from build123d import *

# Parameters (mm, degrees)
SKETCH1_R           = 61.3
BOSS_EXTRUDE1_DEPTH = 1.65
SKETCH2_R           = 55.89
BOSS_EXTRUDE2_DEPTH = 32.735
SKETCH3_R           = 50.86
CUT_EXTRUDE1_DEPTH  = 14.35
SKETCH5_R           = 19.45
BOSS_EXTRUDE3_DEPTH = 0.2
SCALE2_SCALE        = 0.5


with BuildPart() as part:
    # Sketch1 → Boss-Extrude1 (new body)
    with BuildSketch(Plane(origin=(0, 0, 0), x_dir=(1, 0, 0), z_dir=(0, 1, 0))):
        Circle(SKETCH1_R)
    extrude(amount=BOSS_EXTRUDE1_DEPTH)

    # Sketch2 → Boss-Extrude2 (add)
    with BuildSketch(Plane(origin=(0, 1.65, 0), x_dir=(1, 0, 0), z_dir=(0, 1, 0))):
        Circle(SKETCH2_R)
    extrude(amount=BOSS_EXTRUDE2_DEPTH)

    # Sketch3 → Cut-Extrude1 (cut)
    with BuildSketch(Plane.XZ):
        Circle(SKETCH3_R)
    extrude(amount=-CUT_EXTRUDE1_DEPTH, mode=Mode.SUBTRACT)

    # Sketch5 → Boss-Extrude3 (add)
    with BuildSketch(Plane(origin=(0, 34.385, 0), x_dir=(1, 0, 0), z_dir=(0, 1, 0))):
        Circle(SKETCH5_R)
    extrude(amount=BOSS_EXTRUDE3_DEPTH)


with BuildPart() as part_1:
    # Scale2: scaled about (0, 22.178245993, 0)
    add(part.part.scale(SCALE2_SCALE).moved(Location((0, 11.089122997, 0))))


solid = part_1.part
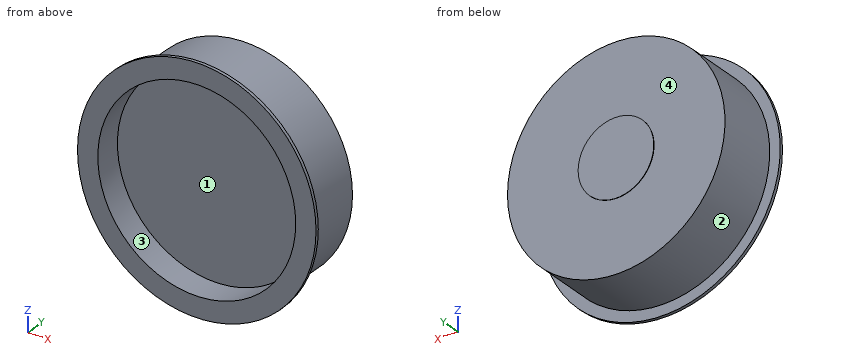
Design review of the part built by this model. Coordinates are the model's own, in mm. Face numbers are marked on the shaded views. Give positions to 0.01 mm unless a question says otherwise; leave off trailing zeros. Order: outer loops, then holes, each group sorted by start corner. A loop starts at its lowest first (then second) coordinate and runs counter-clockwise, first axis right, second up.
1. Add section C-C, the plane y = 17.5. State the section outline as (x, z) points (3 decimals), then the cut area to 3 significant figures.
Solution:
outline: circle Ø55.89 at (0, 0); hole circle Ø50.86 at (0, 0)
area: 422 mm2
2. To check wall thickness, follow L1, parallel to Z at x = 0, y = 13.5 (3 decimals); L2, parallel to Y at x = -3, z = 9; L3, parallel to X at y = 15, z = 17. State the ranges of each line that lie inside material, in increasing order.
Solution:
L1: z = -27.945 to -25.43, 25.43 to 27.945
L2: y = 18.26 to 28.38
L3: x = -22.18 to -18.91, 18.91 to 22.18
3. For pin 1 Ø3 at (x, y) = (-23, 22) entering from +Z; pin 2 Ø2 at (x, z) = (-7.5, 15.5) entering from +Y; pin 3 Ø1.5 at (y, z) = (13.5, -20.5) entering from +X, all flat-tipped, find the tip position at first contact; note any pin that passes through.
Solution:
pin 1: stops at z = 17.85
pin 2: stops at y = 28.28
pin 3: stops at x = 19.77
4. Add section A-A, the plane z = 0. State the section outline as (x, y) points (3 decimals), then the cut area to 3 significant figures.
Solution:
outline: (-30.65, 11.089) - (-25.43, 11.089) - (-25.43, 18.264) - (25.43, 18.264) - (25.43, 11.089) - (30.65, 11.089) - (30.65, 11.914) - (27.945, 11.914) - (27.945, 28.282) - (9.725, 28.282) - (9.725, 28.382) - (-9.725, 28.382) - (-9.725, 28.282) - (-27.945, 28.282) - (-27.945, 11.914) - (-30.65, 11.914) - close
area: 602 mm2
5. Add section D-D, the plane y = 24.5. State the section outline as (x, z) points (3 decimals), then the cut area to 3 significant figures.
Solution:
outline: circle Ø55.89 at (0, 0)
area: 2,450 mm2
6. Mouldability with a two-part tool opening along X and no side actions: class the marked faces 1, 2, 3 and 4 as +X half, -X half, draft (parallel to the pull), parting line (faces both ways), or undercut.
Solution:
face 1: undercut
face 2: parting line
face 3: undercut
face 4: draft
7. Add section B-B, the plane x = 0. State the section outline as (y, z) points (3 decimals), then the cut area to 3 significant figures.
Solution:
outline: (11.089, -30.65) - (11.914, -30.65) - (11.914, -27.945) - (28.282, -27.945) - (28.282, -9.725) - (28.382, -9.725) - (28.382, 9.725) - (28.282, 9.725) - (28.282, 27.945) - (11.914, 27.945) - (11.914, 30.65) - (11.089, 30.65) - (11.089, 25.43) - (18.264, 25.43) - (18.264, -25.43) - (11.089, -25.43) - close
area: 602 mm2
